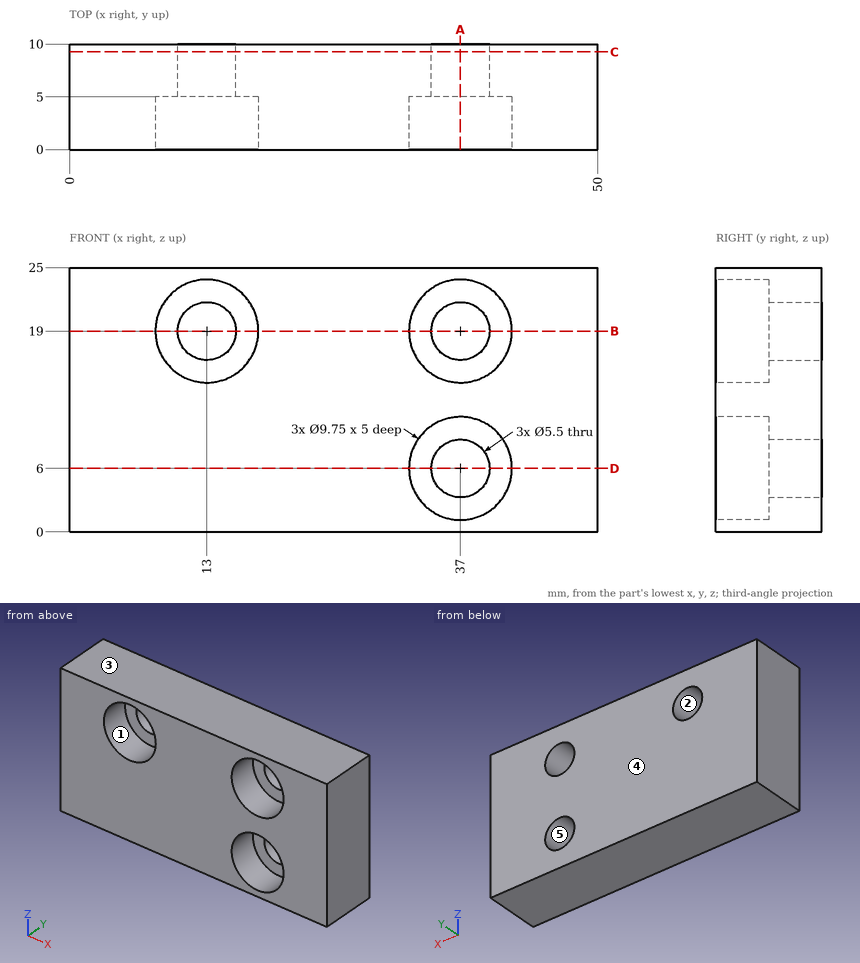
Study the drawing (mm; zero at the part's minimum x, y, z) and answer. A direction names the side the tool comes from. Give positions to 0.01 mm unless a question says otherwise; leave off trailing zeros. Loops run counter-clockwise (first coordinate to the right, second up) from the corner with the lowest first, then second, coordinate; pieces in that order, holes last. Notation, with made-up numbers: (-16, 59) - (28, 59) arc R18 ccw to (28, 63) - close; hole circle Ø1 at (-19, 52.25). An arc over 180 degrees is marked (long way). One line per question, with ' | ' between items.
(1) This flat-tipped pin is pushed along its axis until it touches: pin 1 Ø9 at (x, z) = (37, 19) entering from -Y. Where does it stop, or does it pass through?
Recorded:
pin 1: stops at y = 5
(2) The part is cut by section D-D (z = 6). Write down the section's boundary in (x, y) (3 decimals).
Recorded:
outline: (0, 0) - (32.125, 0) - (32.125, 5) - (34.25, 5) - (34.25, 10) - (0, 10) - close; (39.75, 5) - (41.875, 5) - (41.875, 0) - (50, 0) - (50, 10) - (39.75, 10) - close
(3) Straight lines are drawn through the part: probe 1 along Z at (x, y) = (37, 1.35) (3 decimals); probe 2 along Z at (x, y) = (37, 8.15); probe 3 along X at (y, z) = (8.25, 17.5). For each, find the intervals that lie inside material, in ascending order.
Recorded:
probe 1: z = 0 to 1.125, 10.875 to 14.125, 23.875 to 25 | probe 2: z = 0 to 3.25, 8.75 to 16.25, 21.75 to 25 | probe 3: x = 0 to 10.7, 15.3 to 34.7, 39.3 to 50
(4) The mould has two halves that part along Z. Classify the marked faces 3, 4 and 5: +Z half, -Z half, draft (parallel to the pull), parting line (faces both ways), or undercut.
Recorded:
face 3: +Z half | face 4: draft | face 5: undercut
(5) The part is cut by section B-B (z = 19). Write down the section's boundary in (x, y) (3 decimals), then the cut area to 4 significant figures.
Recorded:
outline: (0, 0) - (8.125, 0) - (8.125, 5) - (10.25, 5) - (10.25, 10) - (0, 10) - close; (15.75, 5) - (17.875, 5) - (17.875, 0) - (32.125, 0) - (32.125, 5) - (34.25, 5) - (34.25, 10) - (15.75, 10) - close; (39.75, 5) - (41.875, 5) - (41.875, 0) - (50, 0) - (50, 10) - (39.75, 10) - close | area: 347.5 mm²
(6) A tool of negligible diameter and unlimited length cuts with its end or side. For the marked faces 1 and 2, from which of +Z, -Z, +X, -X, +Y, -Y can it reach the whole face along a straight path? Write none if from no direction.
Recorded:
face 1: -Y | face 2: +Y, -Y
(7) The part is cut by section A-A (x = 37). Write down the section's boundary in (y, z) (3 decimals), then the cut area to 3 significant figures.
Recorded:
outline: (0, 0) - (10, 0) - (10, 3.25) - (5, 3.25) - (5, 1.125) - (0, 1.125) - close; (0, 10.875) - (5, 10.875) - (5, 8.75) - (10, 8.75) - (10, 16.25) - (5, 16.25) - (5, 14.125) - (0, 14.125) - close; (0, 23.875) - (5, 23.875) - (5, 21.75) - (10, 21.75) - (10, 25) - (0, 25) - close | area: 97.5 mm²
(8) The part is cut by section C-C (y = 9.25). Write down the section's boundary in (x, z), then the cut area to 3 significant figures.
Recorded:
outline: (0, 0) - (50, 0) - (50, 25) - (0, 25) - close; hole circle Ø5.5 at (13, 19); hole circle Ø5.5 at (37, 6); hole circle Ø5.5 at (37, 19) | area: 1,180 mm²
